```python
from build123d import *

# Parameters (mm, degrees)
SKETCH2_R           = 40
SKETCH2_R_2         = 34
BOSS_EXTRUDE1_DEPTH = 129
BOSS_EXTRUDE2_START = -3
BOSS_EXTRUDE2_DEPTH = 3
SKETCH4_R           = 1.75
BOSS_EXTRUDE3_DEPTH = 6
FILLET1_R           = 1
SKETCH5_R           = 1.75
BOSS_EXTRUDE4_DEPTH = 3
CUT_EXTRUDE1_DEPTH  = 45


with BuildPart() as part:
    # Sketch2 → Boss-Extrude1 (new body)
    with BuildSketch(Plane.XY):
        Circle(SKETCH2_R)
        Circle(SKETCH2_R_2, mode=Mode.SUBTRACT)
    extrude(amount=BOSS_EXTRUDE1_DEPTH)

    # Sketch3 → Boss-Extrude2 (add)
    with BuildSketch(Plane.XY.offset(129).offset(BOSS_EXTRUDE2_START)):
        with BuildLine():
            Line((-38.359258991, -11.338749917), (38.359258991, -11.338749917))
            ThreePointArc((38.359258991, -11.338749917), (0, -40), (-38.359258991, -11.338749917))
        make_face()
    extrude(amount=BOSS_EXTRUDE2_DEPTH)

    # Sketch4 → Boss-Extrude3 (add)
    # profile 1 of 2: a face of its own
    with BuildSketch(Plane.XY.offset(68)):
        with BuildLine():
            Line((-35.522508154, -18.388893781), (-43.756797007, -24.37476605))
            ThreePointArc((-43.756797007, -24.37476605), (-45.030952367, -32.827711895), (-36.559912698, -33.975427997))
            Line((-36.559912698, -33.975427997), (-28.469742754, -28.097575474))
            ThreePointArc((-28.469742754, -28.097575474), (-32.362272311, -23.509217998), (-35.522508154, -18.388893781))
        make_face()
        with Locations((-40.230085493, -29.228868016)):
            Circle(SKETCH4_R, mode=Mode.SUBTRACT)
    # profile 2 of 2: a face of its own
    with BuildSketch(Plane.XY.offset(68)):
        with BuildLine():
            Line((28.469742754, -28.097575474), (36.559912698, -33.975427997))
            ThreePointArc((36.559912698, -33.975427997), (45.030952367, -32.827711895), (43.756797007, -24.37476605))
            Line((43.756797007, -24.37476605), (35.522508154, -18.388893781))
            ThreePointArc((35.522508154, -18.388893781), (32.362272311, -23.509217998), (28.469742754, -28.097575474))
        make_face()
        with Locations(Location((40.230085493, -29.228868016, 0), (0, 0, 180))):
            Circle(SKETCH4_R, mode=Mode.SUBTRACT)
    extrude(amount=BOSS_EXTRUDE3_DEPTH)

    # Fillet1
    fillet1_edges = [part.edges().sort_by_distance(p)[0] for p in [
        (-32.362272311, -23.509217998, 74),
        (-32.362272311, -23.509217998, 68),
        (32.362272311, -23.509217998, 74),
        (32.362272311, -23.509217998, 68),
    ]]
    fillet(fillet1_edges, radius=FILLET1_R)

    # Sketch5 → Boss-Extrude4 (add)
    # profile 1 of 2: a face of its own
    with BuildSketch(Plane(origin=(0, 0, 0), x_dir=(-1, 0, 0), z_dir=(0, 0, -1))):
        with BuildLine():
            Line((-39.547439867, 6), (-47.547439867, 6))
            ThreePointArc((-47.547439867, 6), (-53.555028976, 0.287066347), (-48.151184551, -6))
            Line((-48.151184551, -6), (-39.547439867, -6))
            ThreePointArc((-39.547439867, -6), (-40, 0), (-39.547439867, 6))
        make_face()
        with Locations((-47.547439867, -0.015187819)):
            Circle(SKETCH5_R, mode=Mode.SUBTRACT)
    # profile 2 of 2: a face of its own
    with BuildSketch(Plane(origin=(0, 0, 0), x_dir=(-1, 0, 0), z_dir=(0, 0, -1))):
        with BuildLine():
            Line((39.547439867, -6), (48.151184551, -6))
            ThreePointArc((48.151184551, -6), (53.555028976, 0.287066347), (47.547439867, 6))
            Line((47.547439867, 6), (39.547439867, 6))
            ThreePointArc((39.547439867, 6), (40, 0), (39.547439867, -6))
        make_face()
        with Locations(Location((47.547439867, -0.015187819, 0), (0, 0, 180))):
            Circle(SKETCH5_R, mode=Mode.SUBTRACT)
    extrude(amount=-BOSS_EXTRUDE4_DEPTH)

    # Sketch6 → Cut-Extrude1 (cut, symmetric)
    with BuildSketch(Plane.XY.offset(68)):
        with BuildLine():
            Line((-5.405405405, 39.633087092), (-4.594594595, 33.688124028))
            ThreePointArc((-4.594594595, 33.688124028), (0, 34), (4.594594595, 33.688124028))
            Line((4.594594595, 33.688124028), (5.405405405, 39.633087092))
            ThreePointArc((5.405405405, 39.633087092), (0, 40), (-5.405405405, 39.633087092))
        make_face()
        with BuildLine():
            Line((18.922679261, 35.241058577), (16.084277372, 29.95489979))
            ThreePointArc((16.084277372, 29.95489979), (19.984698578, 27.506577809), (23.51848759, 24.553629904))
            Line((23.51848759, 24.553629904), (27.66880893, 28.886623417))
            ThreePointArc((27.66880893, 28.886623417), (23.511410092, 32.360679775), (18.922679261, 35.241058577))
        make_face()
        with BuildLine():
            Line((36.022943608, 17.388143485), (30.619502066, 14.779921962))
            ThreePointArc((30.619502066, 14.779921962), (32.335921554, 10.506577809), (33.45911769, 6.040483704))
            Line((33.45911769, 6.040483704), (39.363667871, 7.106451417))
            ThreePointArc((39.363667871, 7.106451417), (38.042260652, 12.360679775), (36.022943608, 17.388143485))
        make_face()
        with BuildLine():
            Line((39.363667871, -7.106451417), (33.45911769, -6.040483704))
            ThreePointArc((33.45911769, -6.040483704), (32.335921554, -10.506577809), (30.619502066, -14.779921962))
            Line((30.619502066, -14.779921962), (36.022943608, -17.388143485))
            ThreePointArc((36.022943608, -17.388143485), (38.042260652, -12.360679775), (39.363667871, -7.106451417))
        make_face()
        with BuildLine():
            Line((27.66880893, -28.886623417), (23.51848759, -24.553629904))
            ThreePointArc((23.51848759, -24.553629904), (19.984698578, -27.506577809), (16.084277372, -29.95489979))
            Line((16.084277372, -29.95489979), (18.922679261, -35.241058577))
            ThreePointArc((18.922679261, -35.241058577), (23.511410092, -32.360679775), (27.66880893, -28.886623417))
        make_face()
        with BuildLine():
            Line((5.405405405, -39.633087092), (4.594594595, -33.688124028))
            ThreePointArc((4.594594595, -33.688124028), (0, -34), (-4.594594595, -33.688124028))
            Line((-4.594594595, -33.688124028), (-5.405405405, -39.633087092))
            ThreePointArc((-5.405405405, -39.633087092), (0, -40), (5.405405405, -39.633087092))
        make_face()
        with BuildLine():
            Line((-18.922679261, -35.241058577), (-16.084277372, -29.95489979))
            ThreePointArc((-16.084277372, -29.95489979), (-19.984698578, -27.506577809), (-23.51848759, -24.553629904))
            Line((-23.51848759, -24.553629904), (-27.66880893, -28.886623417))
            ThreePointArc((-27.66880893, -28.886623417), (-23.511410092, -32.360679775), (-18.922679261, -35.241058577))
        make_face()
        with BuildLine():
            Line((-36.022943608, -17.388143485), (-30.619502066, -14.779921962))
            ThreePointArc((-30.619502066, -14.779921962), (-32.335921554, -10.506577809), (-33.45911769, -6.040483704))
            Line((-33.45911769, -6.040483704), (-39.363667871, -7.106451417))
            ThreePointArc((-39.363667871, -7.106451417), (-38.042260652, -12.360679775), (-36.022943608, -17.388143485))
        make_face()
        with BuildLine():
            Line((-39.363667871, 7.106451417), (-33.45911769, 6.040483704))
            ThreePointArc((-33.45911769, 6.040483704), (-32.335921554, 10.506577809), (-30.619502066, 14.779921962))
            Line((-30.619502066, 14.779921962), (-36.022943608, 17.388143485))
            ThreePointArc((-36.022943608, 17.388143485), (-38.042260652, 12.360679775), (-39.363667871, 7.106451417))
        make_face()
        with BuildLine():
            Line((-27.66880893, 28.886623417), (-23.51848759, 24.553629904))
            ThreePointArc((-23.51848759, 24.553629904), (-19.984698578, 27.506577809), (-16.084277372, 29.95489979))
            Line((-16.084277372, 29.95489979), (-18.922679261, 35.241058577))
            ThreePointArc((-18.922679261, 35.241058577), (-23.511410092, 32.360679775), (-27.66880893, 28.886623417))
        make_face()
    extrude(amount=CUT_EXTRUDE1_DEPTH, both=True, mode=Mode.SUBTRACT)


solid = part.part
```
Read the model definition and answer for the solid it produces. Units are mm, in the model's axes. A direction names the side the tool comes from. Coordinates: 2 decimals unless noted, no trailing zeros. Loops run counter-clockwise (first coordinate to the right, second up) from the corner with the lowest first, then second, coordinate; pieces in that order, holes last. Notation, with made-up numbers: (12.5, 67.25) -> (66.5, 67.25) arc R12 cw to (66.5, 77.25) -> close; hole circle Ø10 at (82.5, 8.5). An arc over 180 degrees is marked (long way). Return JSON: item names as keys, results as strings.
Item 1: Find the intervals of material crossed by probe 1 along X at (y, z) = (0, 61); probe 2 along Z at (x, y) = (20, -34); probe 3 along Z at (x, y) = (-11.5, -21.5), in increasing order.
Answers:
{"probe 1": "x = -40 to -34, 34 to 40", "probe 2": "z = 0 to 23, 113 to 129", "probe 3": "z = 126 to 129"}
Item 2: Find section C-C (z = 120). Determine the outline of the cut face in (x, y), plus the area to 3 significant figures.
Answers:
{"outline": "circle Ø80 at (0, 0); hole circle Ø68 at (0, 0)", "area": "1,390 mm2"}
Item 3: For a pull along X with two mould halves and no side action, classify faces 1 (the flat face through (-33.283, 16.066, 67.37)), 2 (the flat face through (0, -20, 126)), 3 (the flat face through (-25.565, -26.69, 67.37)), 4 (the cylindrical face through (53.547, 0.415, 1.479)) as +X half, -X half, draft (parallel to the pull), parting line (faces both ways), or undercut.
Answers:
{"face 1": "-X half", "face 2": "undercut", "face 3": "undercut", "face 4": "+X half"}
Item 4: Find section A-A (x = 0). Determine the outline of the cut face in (y, z), plus the area to 3 significant figures.
Answers:
{"outline": "(-40, 0) -> (-34, 0) -> (-34, 23) -> (-40, 23) -> close; (-40, 113) -> (-34, 113) -> (-34, 126) -> (-11.34, 126) -> (-11.34, 129) -> (-40, 129) -> close; (34, 0) -> (40, 0) -> (40, 23) -> (34, 23) -> close; (34, 113) -> (40, 113) -> (40, 129) -> (34, 129) -> close", "area": "536 mm2"}
Item 5: Find section B-B (z = 40). Count the separate pieces of the cut face and the enclosed holes in it, plus the area to 3 significant figures.
Answers:
{"separate pieces": "10", "enclosed holes": "0", "area": "793 mm2"}
Item 6: Flat-ended cylindrical pins translate along their axes: P1, Ø3, axis at x = -33.5, z = 60.5, coming from the +Y side; P2, Ø5.5, axis at x = -23, y = -27.5, coming from the -Z side; P3, Ø10, axis at y = -9.5, z = 59.5, coming from the -X side; P4, Ø10, axis at x = -29.5, z = 112.5, coming from the -Y side. Find the tip coordinate at first contact, or state that the pin passes through.
Answers:
{"P1": "stops at y = 24", "P2": "stops at z = 0", "P3": "stops at x = -39.75", "P4": "stops at y = -31.6"}
Item 7: For faces 5 (the flat face through (-44, 6, 1)), 6 (the flat face through (-17.484, 32.561, 68.63)), 7 (the flat face through (5.006, -36.702, 67.37)), determine the directions among +Z, -Z, +X, -X, +Y, -Y from which every point of the face is accessible in a straight line to the end or side of a thin tool.
Answers:
{"face 5": "+Z, -Z, -X, +Y", "face 6": "-X", "face 7": "-Y"}
Item 8: Find section D-D (x = 21.5). Determine the outline of the cut face in (y, z).
Answers:
{"outline": "(-33.73, 0) -> (-26.34, 0) -> (-26.34, 23) -> (-33.73, 23) -> close; (-33.73, 113) -> (-26.34, 113) -> (-26.34, 126) -> (-11.34, 126) -> (-11.34, 129) -> (-33.73, 129) -> close; (26.34, 0) -> (33.73, 0) -> (33.73, 23) -> (26.34, 23) -> close; (26.34, 113) -> (33.73, 113) -> (33.73, 129) -> (26.34, 129) -> close"}
